```python
from build123d import *

# Parameters (mm, degrees)
SKETCH1_W           = 100
SKETCH1_H           = 116
SKETCH1_R           = 2.2
BOSS_EXTRUDE2_DEPTH = 20
FILLET2_R           = 2
CUT_EXTRUDE7_DEPTH  = 155.45387661
SKETCH22_R          = 1.25
CUT_EXTRUDE12_DEPTH = 118.320075008
CUT_EXTRUDE13_START = -10
CUT_EXTRUDE13_DEPTH = 96
SKETCH26_W          = 24.5
SKETCH26_H          = 20
CUT_EXTRUDE14_DEPTH = 155.45387661
FILLET11_R          = 2


with BuildPart() as part:
    # Sketch1 → Boss-Extrude2 (new body)
    # profile 1 of 5: a face of its own
    with BuildSketch(Plane(origin=(0, 0, 0), x_dir=(1, 0, 0), z_dir=(0, 1, 0))):
        with Locations((50, 0)):
            Rectangle(SKETCH1_W, SKETCH1_H)
        with Locations((97.5, 35)):
            Circle(SKETCH1_R, mode=Mode.SUBTRACT)
        with Locations((97.5, -35)):
            Circle(SKETCH1_R, mode=Mode.SUBTRACT)
        with Locations((75, 35)):
            Circle(SKETCH1_R, mode=Mode.SUBTRACT)
        with Locations((75, -35)):
            Circle(SKETCH1_R, mode=Mode.SUBTRACT)
    # profile 2 of 5: a face of its own
    with BuildSketch(Plane(origin=(0, 0, 0), x_dir=(1, 0, 0), z_dir=(0, 1, 0))):
        with Locations((75, -35)):
            Circle(SKETCH1_R)
    # profile 3 of 5: a face of its own
    with BuildSketch(Plane(origin=(0, 0, 0), x_dir=(1, 0, 0), z_dir=(0, 1, 0))):
        with Locations((97.5, -35)):
            Circle(SKETCH1_R)
    # profile 4 of 5: a face of its own
    with BuildSketch(Plane(origin=(0, 0, 0), x_dir=(1, 0, 0), z_dir=(0, 1, 0))):
        with Locations((75, 35)):
            Circle(SKETCH1_R)
    # profile 5 of 5: a face of its own
    with BuildSketch(Plane(origin=(0, 0, 0), x_dir=(1, 0, 0), z_dir=(0, 1, 0))):
        with Locations((97.5, 35)):
            Circle(SKETCH1_R)
    extrude(amount=-BOSS_EXTRUDE2_DEPTH)

    # Fillet2
    fillet2_edges = [part.edges().sort_by_distance(p)[0] for p in [
        (100, -10, -58),
        (100, -10, 58),
        (0, -10, 58),
        (0, -10, -58),
    ]]
    fillet(fillet2_edges, radius=FILLET2_R)

    # Sketch8 → Cut-Extrude7 (cut, through all)
    with BuildSketch(Plane.XY.offset(58)):
        Polygon((38.788675135, -11), (44.562177826, -11), (59.437822174, -11), (65.211324865, -11), (65.5, -11), (59.437822174, -21.5), (44.562177826, -21.5), (38.5, -11), align=None)
    extrude(amount=-CUT_EXTRUDE7_DEPTH, mode=Mode.SUBTRACT)

    # Sketch22 → Cut-Extrude12 (cut, through all)
    with BuildSketch(Plane(origin=(0, 0, 0), x_dir=(1, 0, 0), z_dir=(0, 1, 0))):
        with Locations(Location((48.25, 0, 0), (0, 0, 270))):
            Circle(SKETCH22_R)
        with Locations(Location((55.75, 0, 0), (0, 0, 270))):
            Circle(SKETCH22_R)
        with Locations(Location((52, 10, 0), (0, 0, 270))):
            Circle(SKETCH22_R)
        with Locations(Location((52, 20, 0), (0, 0, 270))):
            Circle(SKETCH22_R)
        with Locations(Location((52, 35, 0), (0, 0, 270))):
            Circle(SKETCH22_R)
        with Locations(Location((52, -35, 0), (0, 0, 180))):
            Circle(SKETCH22_R)
        with Locations(Location((52, -20, 0), (0, 0, 180))):
            Circle(SKETCH22_R)
        with Locations(Location((52, -10, 0), (0, 0, 180))):
            Circle(SKETCH22_R)
    extrude(amount=-CUT_EXTRUDE12_DEPTH, mode=Mode.SUBTRACT)

    # Sketch24 → Cut-Extrude13 (cut)
    with BuildSketch(Plane(origin=(0, 0, -58), x_dir=(-1, 0, 0), z_dir=(0, 0, -1)).offset(CUT_EXTRUDE13_START)):
        Polygon((-62.035898385, -20), (-67.232050808, -11), (-67.232050808, 0), (-100, 0), (-100, -20), align=None)
    extrude(amount=-CUT_EXTRUDE13_DEPTH, mode=Mode.SUBTRACT)

    # Sketch26 → Cut-Extrude14 (cut, through all)
    with BuildSketch(Plane.XY.offset(58)):
        with Locations((87.75, -10)):
            Rectangle(SKETCH26_W, SKETCH26_H)
    extrude(amount=-CUT_EXTRUDE14_DEPTH, mode=Mode.SUBTRACT)

    # Fillet11
    fillet11_edges = [part.edges().sort_by_distance(p)[0] for p in [
        (67.232050808, -11, 0),
        (75.5, -10, 48),
        (75.5, -10, 58),
        (75.5, -10, -48),
        (75.5, -10, -58),
    ]]
    fillet(fillet11_edges, radius=FILLET11_R)


solid = part.part
```
Here's how the part is built. I have some questions about the finished solid (model axes, mm). A direction names the side the tool comes from. Coordinates: 2 decimals unless noted, no trailing zeros. Order: outer loops, then holes, each group sorted by start corner. A loop starts at its lowest first (then second) coordinate and runs counter-clockwise, first axis right, second up.
Item 1: Thinking about a two-plate mould opening in Y: for faces 1 (the face through (22, -20, -1)), 2 (the face through (75.5, -10, -53)), 3 (the face through (52, -11, 1)), which applies, pulls with the +Y half, pulls with the -Y half, needs draft (parallel to the pull), parting line crosses it, or undercut?
Response values:
face 1: pulls with the -Y half
face 2: needs draft
face 3: undercut
Item 2: If we section it at D-D, the plane z = -22.5: List the corners of the cut face in (x, y) for me, then the cut area to 4 significant figures.
Response values:
outline: (0, -20) - (43.7, -20) - (38.5, -11) - (65.5, -11) - (60.3, -20) - (62.04, -20) - (66.96, -11.46) arc R2 ccw to (67.23, -10.46) - (67.23, 0) - (0, 0) - close
area: 1,125 mm2
Item 3: If we section it at C-C, the plane y = -14.75: List the corners of the cut face in (x, z) for me.
Response values:
outline: (0, -56) arc R2 ccw to (2, -58) - (40.67, -58) - (40.67, 58) - (2, 58) arc R2 ccw to (0, 56) - close; (63.33, -58) - (73.5, -58) arc R2 ccw to (75.5, -56) - (75.5, -50) arc R2 ccw to (73.5, -48) - (65.07, -48) - (65.07, 48) - (73.5, 48) arc R2 ccw to (75.5, 50) - (75.5, 56) arc R2 ccw to (73.5, 58) - (63.33, 58) - close
Item 4: If we section it at B-B, the plane y = -9.25: Give the number of separate pieces and of enclosed holes in the cut face, then the cut area to 3 significant figures.
Response values:
separate pieces: 1
enclosed holes: 8
area: 7,920 mm2
Item 5: Which directions (+Z, -Z, +X, -X, +Y, -Y) give clear straight access to the entire face, cutting with the end or side of a thin tool? Please do faces 4 (the face through (67.232, -5, -1)), 5 (the face through (41.134, -15.563, 0.812)), 6 (the face through (64.466, -15.792, -0.672)).
Response values:
face 4: +X, +Y, -Y
face 5: +Z, -Z
face 6: +X, -Y
Item 6: I need wall thicknesses on probe 1 along X at (y, z) = (-3.5, 0); probe 2 along Z at (x, y) = (70.5, -14); probe 3 along X at (y, z) = (-8.5, -10). Which ranges of each line are inside material? Lowest first, please.
Response values:
probe 1: x = 0 to 47, 49.5 to 54.5, 57 to 67.23
probe 2: z = -58 to -48, 48 to 58
probe 3: x = 0 to 50.75, 53.25 to 67.23
Item 7: I'm going to push flat-ended pins straight in: pin 1 Ø2 at (x, z) = (52, -20) entering from -Y; pin 2 Ø4 at (x, z) = (55.75, 0) entering from -Y; pin 3 Ø8 at (y, z) = (-7.5, 36.5) entering from +X; pin 4 Ø5 at (x, z) = (66, 45) entering from -Y. Where does each tip first touch, or does it pass through?
Response values:
pin 1: passes through
pin 2: stops at y = -11
pin 3: stops at x = 67.23
pin 4: stops at y = -17.46
Item 8: If we section it at A-A, the plane z = -35: List the corners of the cut face in (x, y) for me, then the cut area to 3 significant figures.
Response values:
outline: (0, -20) - (43.7, -20) - (38.5, -11) - (50.75, -11) - (50.75, 0) - (0, 0) - close; (53.25, -11) - (65.5, -11) - (60.3, -20) - (62.04, -20) - (66.96, -11.46) arc R2 ccw to (67.23, -10.46) - (67.23, 0) - (53.25, 0) - close
area: 1,100 mm2
